Can you work these out from the drawing? Everything is in mm from the part's minimum corner. Round coordinates to 2 decimals unless told otherwise and drop trailing zeros. Order: outer loops, then holes, each group sorted by start corner. A loop starts at its lowest first (then second) coordinate and runs counter-clockwise, first axis right, second up. Notation, with made-up numbers: M 66,-14.5 L 119,-14.5 A32 cw 119,13.5 Z; hole C 10.5,-33 d5. An arc over 180 degrees is marked long. Answer as a JSON object with one key per item and string values. Group by question number.
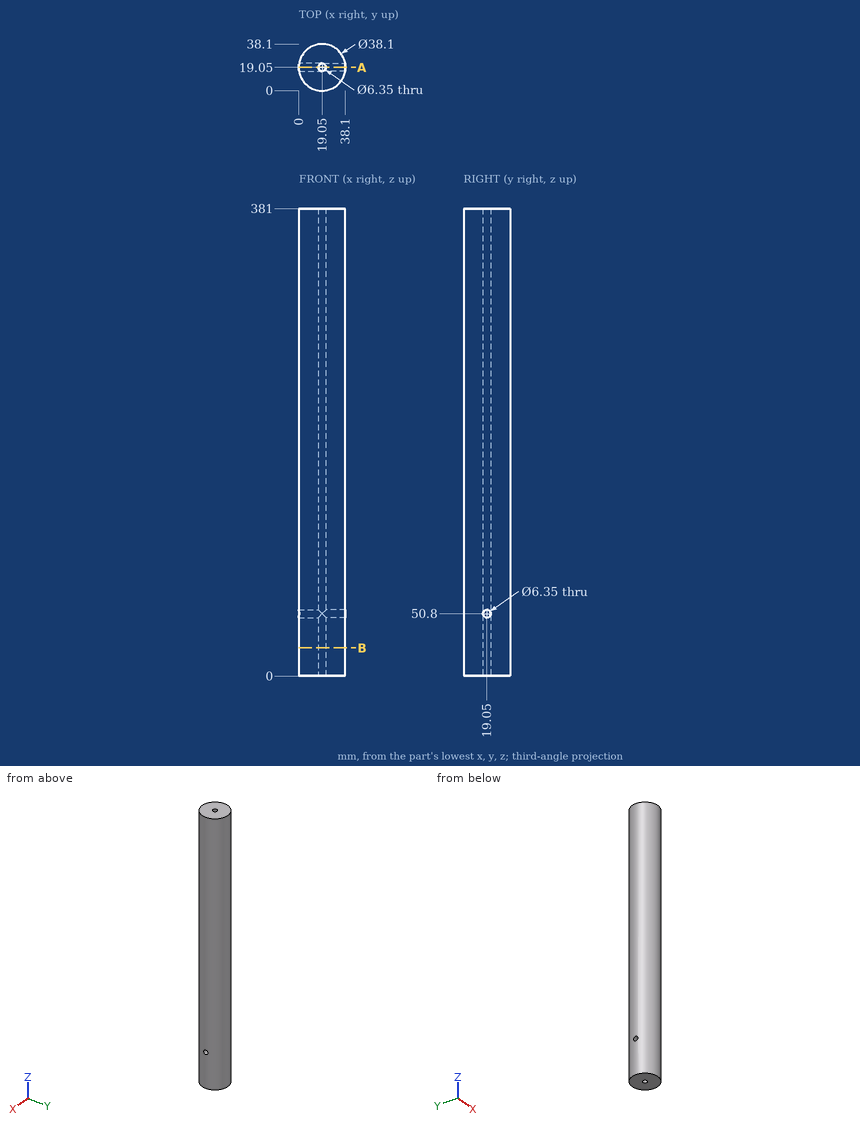
Item 1: I need wall thicknesses on line 1 (Y direction, x = 19, z = 319); line 2 (Y direction, x = 21.5, z = 204.5). Which ranges of each line are inside material? Lowest first, please.
Item 2: I'm going to push flat-ended pins straight in: pin 1 Ø4 at (y, z) = (23.5, 259.5) entering from -X; pin 2 Ø5 at (x, z) = (12.5, 197.5) entering from -Y; pin 3 Ø5 at (y, z) = (25, 223.5) entering from +X (3 decimals). Where does each tip first touch, or does it pass through?
Item 3: Suppose I cut it at A-A, the plane y = 19.05. Write out the boundary of the cut face in (x, z) (3 decimals).
Item 4: Suppose I cut it at B-B, the plane z = 23. Write out the boundary of the cut face in (x, y) (3 decimals), and give its area (3 significant figures).
Computed:
{
 "1": {"line 1": "y = 0 to 15.88, 22.22 to 38.1", "line 2": "y = 0.16 to 17.03, 21.07 to 37.94"},
 "2": {"pin 1": "stops at x = 0.16", "pin 2": "stops at y = 0.44", "pin 3": "stops at x = 37.785"},
 "3": {"outline": "M 0,0 L 15.875,0 L 15.875,47.625 L 0,47.625 Z; M 0,53.975 L 15.875,53.975 L 15.875,381 L 0,381 Z; M 22.225,0 L 38.1,0 L 38.1,47.625 L 22.225,47.625 Z; M 22.225,53.975 L 38.1,53.975 L 38.1,381 L 22.225,381 Z"},
 "4": {"outline": "C 19.05,19.05 d38.1; hole C 19.05,19.05 d6.35", "area": "1,110 mm^2"}
}
